Model file for the job. Use its own axes, mm. A direction names the side the tool comes from. Coordinates: 2 decimals unless noted, no trailing zeros.
Autodesk Inventor part; units mm, degrees
ref_plane "Work Plane1" through (40, 33.3148, 0) normal (1, 0, 0) x (0, 1, 0)
ref_plane "XZ Plane" through (0, 0, 0) normal (0, 1, 0) x (-1, 0, 0)
ref_plane "XY Plane" through (0, 0, 0) normal (0, 0, 1) x (1, 0, 0)
sketch "Sketch1" plane through (0, 0, 0) normal (0, 0, 1) x (1, 0, 0)
  line L0 (0, 30.8148) -> (40, 30.8148)
  line L1 (40, 30.8148) -> (40, 35.8148)
  line L2 (0, 30.8148) -> (0, 0)
  line L3 (0, 0) -> (140, 0)
  arc A0 (140, 0) -> (40, 35.8148) centre (40.5629, -120.1278) ccw
  dimension "d0" = 40
  dimension "d1" = 5
  dimension "d2" = 140
revolve "Revolution1" add sketch "Sketch1" angle 360 about axis through (0, 30.8148, 0) along (0, -1, 0)
shell "Shell1" thickness 3 removed faces 1 at (22.2847, 0, -49.1516)
sketch "Sketch2" plane through (0, 30.8148, 0) normal (0, 1, 0) x (1, 0, 0)
  circle A0 centre (0, 0) radius 37
  dimension "d5" = 74
extrude "Extrusion1" cut sketch "Sketch2" against normal through all
ref_plane "Work Plane1" through (40, 33.3148, 0) normal (1, 0, 0) x (0, 1, 0)
sketch "Sketch4" plane through (40, 33.3148, 0) normal (1, 0, 0) x (0, 1, 0)
  line L0 (1, -1.0043) -> (-1, -1.0043)
  line L1 (-1, -1.0043) -> (-1, 0.9957)
  line L2 (-1, 0.9957) -> (1, 0.9957)
  line L3 (1, 0.9957) -> (1, -1.0043)
  line L4 (-2.5, 40) -> (-2.5, -40)
  point P0 (-33.3148, 0)
  dimension "d8" = 2
  dimension "d9" = 2
  dimension "d10" = 1.5
extrude "Extrusion2" add sketch "Sketch4" against normal blind 2
pattern_circular "Circular Pattern1" count 2 over 360 about axis through (0, 30.8148, 0) along (0, -1, 0) of "Extrusion2"
equation "\"d9\" = d8"
properties part number "topplock"
Q1. Mould opens along Z. For faces 3 (the cylindrical face through (-8.67, 33.35, 39.05)), 4 (the flat face through (-115, 0, 73)) say: +Z half, -Z half, draft (parallel to the pull), parting line (faces both ways), or undercut.
Answers:
face 3: undercut
face 4: draft
Q2. Flat gauge pins, fed straight in: P1, Ø4, axis at x = -93.5, z = 17.5, coming from the -Y side; P2, Ø12, axis at x = 44.5, z = 47.5, coming from the +Y side; P3, Ø3, axis at x = 0, y = 23.5, coming from the +Z side. Where does each tip first touch, or does it go through?
Answers:
P1: stops at y = 21.97
P2: stops at y = 34.71
P3: stops at z = 104.74
Q3. Which spindle directions (+Z, -Z, +X, -X, +Y, -Y) get a long thin tool onto all of the face, cutting with end or side? Do faces 1 (the cylindrical face through (-8.02, 29.34, 36.12)), 2 (the cylindrical face through (-5.598, 30.34, -42.634)). Say none if no direction does.
Answers:
face 1: +Y, -Y
face 2: -Y
Q4. Drill centre lines: line 1 (X direction, y = 17.5, z = -24); line 2 (X direction, y = 4.5, z = 82.5); line 3 (Z direction, x = -15, y = 12.5). Where is each one in solid material? Low to high.
Answers:
line 1: x = -111.33 to -104.55, 104.55 to 111.33
line 2: x = -105.97 to -99.45, 99.45 to 105.97
line 3: z = -121.67 to -115.76, 115.76 to 121.67
